For this review, take the finished solid that the model builds, in its own axes (mm). A direction names the side the tool comes from. Give positions to 0.01 mm unless a question says otherwise; leave off trailing zeros. Loops run counter-clockwise (first coordinate to the right, second up) from the corner with the lowest first, then second, coordinate; pieces in that order, holes last.
Autodesk Inventor part; units mm, degrees
ref_plane "YZ Plane" through (0, 0, 0) normal (1, 0, 0) x (0, 1, 0)
ref_plane "XZ Plane" through (0, 0, 0) normal (0, 1, 0) x (-1, 0, 0)
ref_plane "XY Plane" through (0, 0, 0) normal (0, 0, 1) x (1, 0, 0)
sketch "Sketch1" plane through (0, 0, 0) normal (0, 0, 1) x (1, 0, 0)
  line L0 (0, 66) -> (0, -66) construction
  line L1 (-17, 66) -> (-17, -66)
  line L2 (17, -66) -> (17, 66)
  arc A0 (17, 66) -> (-17, 66) centre (0, 66) ccw
  arc A1 (-17, -66) -> (17, -66) centre (0, -66) ccw
  circle A2 centre (0, -66) radius 1.1
  circle A3 centre (0, 66) radius 11.1
  point P0 (0, 0)
  dimension "d0" = 66
  dimension "d1" = 34
  dimension "d2" = 2.2
  dimension "d3" = 22.2
  dimension "d40" = 17
extrude "Extrusion1" add sketch "Sketch1" along normal blind 8
sketch "Sketch2" plane through (0, 0, 8) normal (0, 0, 1) x (1, 0, 0)
  arc A0 (-17, -66) -> (17, -66) centre (0, -66) ccw
  line L0 (17, -66) -> (17, 66)
  arc A1 (17, 66) -> (-17, 66) centre (0, 66) ccw
  line L1 (-17, 66) -> (-17, -66)
  circle A2 centre (0, 66) radius 11.1
  circle A3 centre (0, -66) radius 1.1
  circle A4 centre (0, -66) radius 4.1
  circle A5 centre (0, 66) radius 4.1
  point P0 (0, 0)
  dimension "d6" = 8.2
  dimension "d12" = 8.2
extrude "Extrusion2" add sketch "Sketch2" along normal blind 10 contours L1 A1 L0 A0 | A2
sketch "Sketch3" plane through (0, 0, 18) normal (0, 0, 1) x (1, 0, 0)
  line L0 (17, -66) -> (17, 66)
  arc A0 (17, 66) -> (-17, 66) centre (0, 66) ccw
  line L1 (-17, 66) -> (-17, -66)
  arc A1 (-17, -66) -> (17, -66) centre (0, -66) ccw
  circle A2 centre (0, -66) radius 4.1
  line L2 (0, 49) -> (0, -56) construction
  line L3 (-12, 37) -> (-12, -44)
  line L4 (12, -44) -> (12, 37)
  arc A3 (12, 37) -> (-12, 37) centre (0, 37) ccw
  arc A4 (-12, -44) -> (12, -44) centre (0, -44) ccw
  line L5 (-12, -44) -> (-12, -17)
  line L6 (12, 37) -> (12, 10)
  line L7 (12, -44) -> (-12, -17)
  line L8 (-12, -17) -> (12, 10)
  line L9 (12, 10) -> (-12, 37)
  line L10 (13.1211, 10.9965) -> (-11.8222, 39.0578)
  line L11 (10.8789, 9.0035) -> (-13.1211, 36.0035)
  line L12 (-13.1211, -16.0035) -> (10.8789, 10.9965)
  line L13 (11.8222, -46.0578) -> (-13.1211, -17.9965)
  line L14 (13.1211, -43.0035) -> (-10.8789, -16.0035)
  line L15 (-10.8789, -17.9965) -> (13.1211, 9.0035)
  point P0 (0, -3.5)
  point P1 (-12, -19.2578)
  point P2 (12, 7.7422)
  point P3 (-9.9931, -17)
  point P4 (12, -41.7422)
  point P5 (-12, -14.7422)
  point P6 (9.9931, 10)
  point P7 (-12, 34.7422)
  point P8 (12, 12.2578)
  dimension "d47" = 105
  dimension "d48" = 24
  dimension "d49" = 27
  dimension "d50" = 27
  dimension "d51" = 1.5
  dimension "d52" = 1.5
  dimension "d53" = 1.5
  dimension "d54" = 1.5
  dimension "d55" = 1.5
  dimension "d56" = 1.5
extrude "Extrusion3" cut sketch "Sketch3" against normal up to next contours L11 L12 L3 | A3 L4 L10 | L4 L14 L15 | L13 A4 L3
sketch "Sketch6" plane through (0, -66, 8) normal (0, 0, 1) x (1, 0, 0)
  circle A0 centre (0, 0) radius 4.1
  circle A1 centre (0, 0) radius 1.1
  point P0 (0, 66)
extrude "Extrusion6" cut sketch "Sketch6" against normal up to next contours A0 | A1
fillet "Fillet3" radius 2 10 edges at (-12, 34.7422, 9) (12, 12.2578, 9) (9.9931, 10, 9) (12, 7.7422, 9) (-12, -14.7422, 9) (-9.9931, -17, 9) (-12, -19.2578, 9) (12, -41.7422, 9) (11.8222, -46.0578, 9) (-11.8222, 39.0578, 9)
equation "\"d12\" = d6"
equation "\"d50\" = d49"
properties part number "CodoTrasero" material "PLA"
Item 1: Take a section at B-B on y = -54. Give the boundary of the cut face in (x, z).
Answer:
outline: (-17, 0) - (-6.63, 0) - (-6.63, 18) - (-17, 18) - close; (6.63, 0) - (17, 0) - (17, 18) - (6.63, 18) - close
Item 2: Take a section at A-A on z = 15. Give the boundary of the cut face in (x, y), and give its area (3 significant figures).
Answer:
outline: (-17, -66) arc R17 ccw to (17, -66) - (17, 66) arc R17 ccw to (-17, 66) - close; hole (-12, -44) arc R12 ccw to (11.58, -47.15) arc R2 ccw to (11.14, -45.3) - (-8.51, -23.19) arc R2 ccw to (-12, -24.52) - close; hole (-12, -9.48) arc R2 ccw to (-8.51, -10.81) - (8.81, 8.67) arc R2 ccw to (8.81, 11.33) - (-8.51, 30.81) arc R2 ccw to (-12, 29.48) - close; hole (-11.58, 40.15) arc R2 ccw to (-11.14, 38.3) - (8.51, 16.19) arc R2 ccw to (12, 17.52) - (12, 37) arc R12 ccw to start; hole (-8.81, -18.33) - (8.51, -37.81) arc R2 ccw to (12, -36.48) - (12, 2.48) arc R2 ccw to (8.51, 3.81) - (-8.81, -15.67) arc R2 ccw to start; hole circle Ø8.2 at (0, -66); hole circle Ø8.2 at (0, 66)
area: 3,250 mm2
Item 3: Tool access review of faces 4 (the cylindrical face through (-9.317, -17.02, 8.874)), 5 (the cylindrical face through (-1.445, 54.994, 3.944)), 6 (the flat face through (4, 1, 18)): name each direction out of +Z, -Z, +X, -X, +Y, -Y from which nothing blocks a thin tool from reaching the whole face with its end or side.
Answer:
face 4: +Z, -Z
face 5: -Z
face 6: +Z, +X, -X, +Y, -Y
Item 4: For L1, parallel to Y at x = 6, z = 15.5; L2, parallel to Y at x = -9, z = 13.5; L3, parallel to X at y = -6, z = 1, list the stretches that pass through material, from the lowest coordinate up.
Answer:
L1: y = -81.91 to -54.39, -39.51 to -34.99, 0.99 to 5.51, 14.49 to 19.01, 47.39 to 81.91
L2: y = -80.42 to -51.94, -22.79 to -18.08, -15.92 to -11.21, 31.21 to 35.88, 44.94 to 80.42
L3: x = -17 to -12, -4.23 to -0.22, 12 to 17
Item 5: Take a section at C-C on x = 1. State how many separate pieces and enclosed holes the cut face has, and give its area (3 significant figures).
Answer:
separate pieces: 7
enclosed holes: 0
area: 943 mm2
Item 6: The part is to be moulded in two halves that separate along Y. For faces 1 (the cylindrical face through (0, 83, 9)), 2 (the flat face through (0.275, 20.933, 9.126)), 3 (the flat face through (17, -1, 9)), say which applies: released by +Y, released by -Y, zero draft, split by the parting line, or undercut.
Answer:
face 1: released by +Y
face 2: undercut
face 3: zero draft
Item 7: Take a section at D-D on z = 3.75. Give the boundary of the cut face in (x, y), and give its area (3 significant figures).
Answer:
outline: (-17, -66) arc R17 ccw to (17, -66) - (17, 66) arc R17 ccw to (-17, 66) - close; hole (-12, -44) arc R12 ccw to (11.58, -47.15) arc R2 ccw to (11.14, -45.3) - (-8.51, -23.19) arc R2 ccw to (-12, -24.52) - close; hole (-12, -9.48) arc R2 ccw to (-8.51, -10.81) - (8.81, 8.67) arc R2 ccw to (8.81, 11.33) - (-8.51, 30.81) arc R2 ccw to (-12, 29.48) - close; hole (-11.58, 40.15) arc R2 ccw to (-11.14, 38.3) - (8.51, 16.19) arc R2 ccw to (12, 17.52) - (12, 37) arc R12 ccw to start; hole circle Ø22.2 at (0, 66); hole (-8.81, -18.33) - (8.51, -37.81) arc R2 ccw to (12, -36.48) - (12, 2.48) arc R2 ccw to (8.51, 3.81) - (-8.81, -15.67) arc R2 ccw to start; hole circle Ø8.2 at (0, -66)
area: 2,910 mm2
Item 8: Clearance check with flat-ended pins moving along their axes: pin 1 Ø1.5 at (x, z) = (-5, 12) entering from -Y; pin 2 Ø6.5 at (x, y) = (4, 62.5) entering from -Z; pin 3 Ø7.5 at (x, y) = (0, -66) entering from +Z. State where each tip first meets the part, or that it passes through.
Answer:
pin 1: stops at y = -82.46
pin 2: stops at z = 8
pin 3: passes through
